Geometry check sheet. Reference: the model listing, model coordinates, mm. Face numbers are marked on the shaded views. Give positions to 0.01 mm unless a question says otherwise; leave off trailing zeros. Loops run counter-clockwise (first coordinate to the right, second up) from the corner with the lowest first, then second, coordinate; pieces in that order, holes last. Notation, with made-up numbers: (74.25, -6) -> (98.25, -6) arc R17 cw to (98.25, 20) -> close; hole circle Ø8 at (-19.5, -27.75). An arc over 180 degrees is marked (long way). One line per question, with ' | ' between items.
from build123d import *

# Parameters (mm, degrees)
BOSS_EXTRUDE1_DEPTH     = 279.4
CONVERT_SOLID1_START    = -279.4
CONVERT_SOLID1_DEPTH    = 558.8
CONVERT_SOLID1_2_DEPTH  = 558.8
CUT_EXTRUDE1_DEPTH      = 586.091506768
EDGE_FLANGE1_DEPTH      = 412.817360463
EDGE_FLANGE1_BEND_DEPTH = 412.817360463
SKETCH12_R              = 7.9375
CUT_EXTRUDE2_DEPTH      = 592.463463584


# Read off the part's stored shape, not the designer's step: Convert-Solid1
# Sheet-metal steps are written as plain solids
with BuildPart() as part:
    # Sketch3 → Boss-Extrude1 (new, symmetric)
    with BuildSketch(Plane(origin=(0, 0, 0), x_dir=(0, 0, -1), z_dir=(1, 0, 0))):
        Polygon((-477.990419123, 101.6), (-503.390419123, 101.6), (-503.390419123, 104.14), (-477.723454365, 104.14), (-118.969509086, 27.884494906), (-119.497604781, 25.4), align=None)
    extrude(amount=BOSS_EXTRUDE1_DEPTH, both=True)

    # Convert-Solid1 outline → Convert-Solid1 (cut)
    with BuildSketch(Plane.YZ.offset(CONVERT_SOLID1_START)):
        with BuildLine():
            Line((104.14, 477.723454365), (104.14, 478.257383881))
            ThreePointArc((104.14, 478.257383881), (104.112171228, 477.726379287), (104.028989812, 477.201192491))
            Line((104.028989812, 477.201192491), (104.14, 477.723454365))
        make_face()
    extrude(amount=CONVERT_SOLID1_DEPTH, mode=Mode.SUBTRACT)

    # Convert-Solid1 2 outline → Convert-Solid1 2 (add)
    with BuildSketch(Plane.YZ.offset(CONVERT_SOLID1_START)):
        with BuildLine():
            Line((101.6, 477.990419123), (101.6, 478.257383881))
            ThreePointArc((101.6, 478.257383881), (101.586085614, 477.991881584), (101.544494906, 477.729288186))
            Line((101.544494906, 477.729288186), (101.6, 477.990419123))
        make_face()
    extrude(amount=CONVERT_SOLID1_2_DEPTH)

    # Sketch8 → Cut-Extrude1 (cut, through all)
    with BuildSketch(Plane(origin=(0, 2.484494906, -0.528095695), x_dir=(1, 0, 0), z_dir=(0, 0.978147600733807, -0.20791169081775257))):
        Polygon((279.4, -488.402044668), (88.9, -122.167252357), (279.4, -122.167252357), align=None)
        Polygon((-88.9, -122.167252357), (-279.4, -488.402044668), (-279.4, -122.167252357), align=None)
    extrude(amount=-CUT_EXTRUDE1_DEPTH, mode=Mode.SUBTRACT)

    # Edge-Flange1 section (across the edge) → Edge-Flange1 (add)
    with BuildSketch(Plane(origin=(281.653384818, 103.785293108, 476.054689643), x_dir=(-0.8871593769725215, 0.09594358400128161, 0.4513790741037036), z_dir=(-0.46146315112880654, -0.18445080609118086, -0.8677728160541711))):
        with BuildLine():
            Line((-2.54, 2.54), (-2.54, 22.86))
            Line((-2.54, 22.86), (0, 22.86))
            Line((0, 22.86), (0, 2.54))
            ThreePointArc((0, 2.54), (0.743948776, 0.743948776), (2.54, 0))
            Line((2.54, 0), (2.54, -2.54))
            ThreePointArc((2.54, -2.54), (-1.052102448, -1.052102448), (-2.54, 2.54))
        make_face()
    extrude(amount=EDGE_FLANGE1_DEPTH)

    # Edge-Flange1 section 2 (across the edge) → Edge-Flange1 bend (add)
    with BuildSketch(Plane(origin=(-91.153384818, 27.640798203, 117.823006238), x_dir=(0.8871593769725281, 0.09594358400127896, 0.4513790741036911), z_dir=(-0.46146315112879377, 0.18445080609118228, 0.8677728160541774))):
        with BuildLine():
            Line((-2.54, 2.54), (-2.54, 22.86))
            Line((-2.54, 22.86), (0, 22.86))
            Line((0, 22.86), (0, 2.54))
            ThreePointArc((0, 2.54), (0.743948776, 0.743948776), (2.54, 0))
            Line((2.54, 0), (2.54, -2.54))
            ThreePointArc((2.54, -2.54), (-1.052102448, -1.052102448), (-2.54, 2.54))
        make_face()
    extrude(amount=EDGE_FLANGE1_BEND_DEPTH)

    # Sketch12 → Cut-Extrude2 (cut, symmetric)
    with BuildSketch(Plane(origin=(0, 2.484494906, -0.528095695), x_dir=(1, 0, 0), z_dir=(0, 0.9781476007338071, -0.2079116908177526))):
        with Locations(Location((217.989950501, -411.623430458, 0), (0, 0, 90))):
            Circle(SKETCH12_R)
        with Locations(Location((77.335982037, -141.217252357, 0), (0, 0, 90))):
            Circle(SKETCH12_R)
    cut_extrude2 = extrude(amount=CUT_EXTRUDE2_DEPTH, both=True, mode=Mode.SUBTRACT)

    # Mirror8: Cut-Extrude2 across plane
    add(cut_extrude2.mirror(Plane(origin=(0, 0, 0), x_dir=(0, 0, 1), z_dir=(1, 0, 0))), mode=Mode.SUBTRACT)


solid = part.part
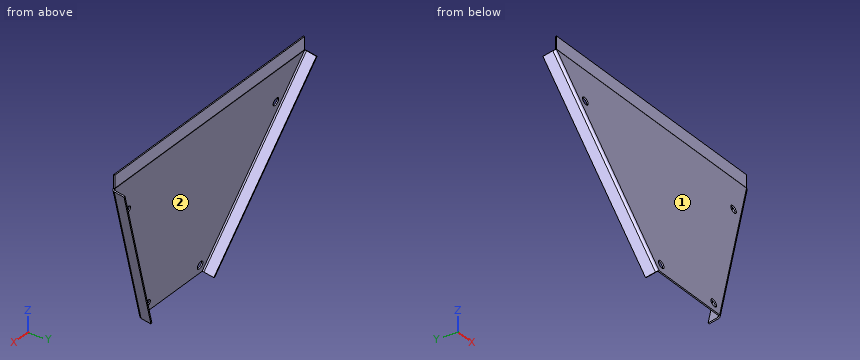
Item 1: Scan lines: probe 1 along X at (y, z) = (77.5, 267.5); probe 2 along Y at (x, z) = (15.5, 181); probe 3 along Y at (x, z) = (170, 276.5). Record each from-to range of solid material in increasing order.
Result:
probe 1: -175.56 to -172.7, 172.7 to 175.56 | probe 2: 38.47 to 41.07 | probe 3: 58.77 to 61.37
Item 2: Sectioned sample at A-A (y = 113.5). Record the cut outline in (x, z), plus the area to 3 significant figures.
Result:
outline: (-283.91, 472.79) -> (-252.88, 411.81) -> (-250.02, 411.81) -> (-281.65, 473.99) -> close; (250.02, 411.81) -> (252.88, 411.81) -> (283.91, 472.79) -> (281.65, 473.99) -> close | area: 353 mm2
Item 3: Depth check by flat-ended pin: pin 1 Ø2 at (y, z) = (102.5, 489) entering from +X; pin 2 Ø7.5 at (x, z) = (83, 486) entering from +Y; pin 3 Ø3 at (y, z) = (102.5, 487.5) entering from -X. Enter the tip coordinate at first touch or a pass-through.
Result:
pin 1: x = 279.4 | pin 2: y = 104.14 | pin 3: x = -279.4
Item 4: Sectioned sample at B-B (x = -13.5). Record the cut outline in (y, z).
Result:
outline: (25.4, 119.5) -> (27.88, 118.97) -> (104.03, 477.2) arc R5.08 ccw to (104.14, 478.26) -> (104.14, 503.39) -> (101.6, 503.39) -> (101.6, 478.26) arc R2.54 cw to (101.54, 477.73) -> close
Item 5: Release check for a two-part mould opening along X. For the marked faces 1 and 2 record: pulls with the +X half, pulls with the -X half, needs draft (parallel to the pull), parting line crosses it, or undercut.
Result:
face 1: needs draft | face 2: undercut
